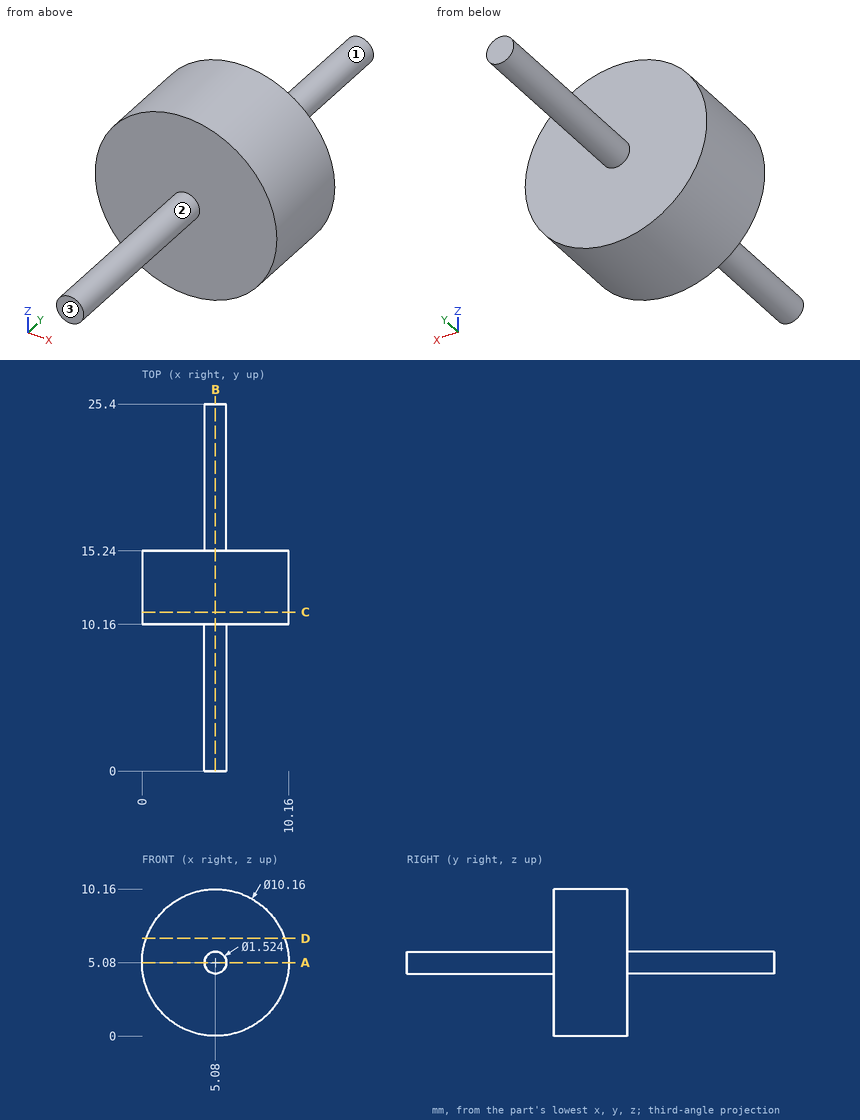
Study the drawing (mm; zero at the part's minimum x, y, z) and answer. A direction names the side the tool comes from. Coordinates: 2 decimals unless noted, no trailing zeros. Write each loop counter-clockwise with the first axis right and the second up, starting at its lowest first coordinate (ties: lowest second). Pieces come first, ordered by that corner, then holes. Notation, with made-up numbers: (18.5, 29) - (61.5, 29) arc R31 ccw to (61.5, 63) - close; hole circle Ø6 at (31, -5.5). An arc over 180 degrees is marked (long way). Answer as a JSON object with one key per item and string values.
Q1. Find section C-C (y = 11). Write down the section's boundary in (x, z), plus the area to 3 significant figures.
Results list:
{"outline": "circle Ø10.16 at (5.08, 5.08)", "area": "81.1 mm^2"}
Q2. Consider L1, parallel to Y at x = 3.5, z = 6.25; L2, parallel to X at y = 18, z = 5; L3, parallel to X at y = 14, z = 7. Determine where each line is inside the solid, lowest interval first. Write a range as from..to.
Results list:
{"L1": "y = 10.16..15.24", "L2": "x = 4.32..5.84", "L3": "x = 0.38..9.78"}
Q3. Which of the six approach directions +Z, -Z, +X, -X, +Y, -Y give full straight-line access (tool end or side, diameter ignored) to the marked faces 1, 2 and 3?
Results list:
{"face 1": "+Y", "face 2": "-Y", "face 3": "+Z, -Z, +X, -X, -Y"}
Q4. Given pin 1 Ø6 at (x, y) = (2, 5) entering from +Z; pin 2 Ø3 at (x, y) = (2, 14) entering from -Z; pin 3 Ø3 at (x, z) = (4.5, 3.5) entering from -Y; pin 4 Ø4 at (x, z) = (3, 7.5) entering from +Y, each flat-ended and moving along its own axis, determine where each tip first touches the part or whether it passes through.
Results list:
{"pin 1": "stops at z = 5.84", "pin 2": "stops at z = 0.25", "pin 3": "stops at y = 0", "pin 4": "stops at y = 15.24"}
Q5. Find section B-B (x = 5.08). Write down the section's boundary in (y, z), plus the area to 3 significant figures.
Results list:
{"outline": "(0, 4.32) - (10.16, 4.32) - (10.16, 0) - (15.24, 0) - (15.24, 4.32) - (25.4, 4.32) - (25.4, 5.84) - (15.24, 5.84) - (15.24, 10.16) - (10.16, 10.16) - (10.16, 5.84) - (0, 5.84) - close", "area": "82.6 mm^2"}
Q6. Find section A-A (z = 5.08). Write down the section's boundary in (x, y), plus the area to 3 significant figures.
Results list:
{"outline": "(0, 10.16) - (4.32, 10.16) - (4.32, 0) - (5.84, 0) - (5.84, 10.16) - (10.16, 10.16) - (10.16, 15.24) - (5.84, 15.24) - (5.84, 25.4) - (4.32, 25.4) - (4.32, 15.24) - (0, 15.24) - close", "area": "82.6 mm^2"}
Q7. Find section D-D (z = 6.75). Write down the section's boundary in (x, y), plus the area to 3 significant figures.
Results list:
{"outline": "(0.28, 10.16) - (9.88, 10.16) - (9.88, 15.24) - (0.28, 15.24) - close", "area": "48.7 mm^2"}
